Geometry: final body of the model. Coordinates: model frame, mm. A direction names the side the tool comes from. Give positions to 0.01 mm unless a question says otherwise; leave off trailing zeros. Loops run counter-clockwise (first coordinate to the right, second up) from the corner with the lowest first, then second, coordinate; pieces in that order, holes last. Notation, with made-up numbers: (61.5, 47) - (100.5, 47) arc R20 ccw to (100.5, 82) - close; hole circle Ø9 at (35, 1.25). An arc over 180 degrees is marked (long way). Answer in a Markdown table with one row per item.
from build123d import *

# Parameters (mm, degrees)
BOSS_EXTRUDE1_DEPTH = 265.3
SKETCH2_W           = 10
SKETCH2_H           = 44
BOSS_EXTRUDE2_DEPTH = 10
SKETCH3_W           = 381.110289958
SKETCH3_H           = 88.245673433
CUT_EXTRUDE1_DEPTH  = 27
SKETCH4_W           = 28
SKETCH4_H           = 7
BOSS_EXTRUDE3_DEPTH = 7


with BuildPart() as part:
    # Sketch1 → Boss-Extrude1 (new body)
    with BuildSketch(Plane(origin=(0, 0, 0), x_dir=(1, 0, 0), z_dir=(0, 1, 0))):
        Polygon((-51.505795374, 37), (-51.505795374, -18), (-41.505795374, -18), (-41.505795374, -37), (-38.505795374, -37), (-38.505795374, -22), (-35.205795374, -22), (-35.205795374, -37), (-32.205795374, -37), (-32.205795374, 37), align=None)
    extrude(amount=BOSS_EXTRUDE1_DEPTH)

    # Sketch2 → Boss-Extrude2 (add)
    with BuildSketch(Plane(origin=(0, 265.3, 0), x_dir=(1, 0, 0), z_dir=(0, 1, 0))):
        with Locations((-41.505795374, 15)):
            Rectangle(SKETCH2_W, SKETCH2_H)
    extrude(amount=BOSS_EXTRUDE2_DEPTH)

    # Sketch3 → Cut-Extrude1 (cut)
    with BuildSketch(Plane(origin=(-16.102897687, -16.102897687, 0), x_dir=(0, 0, -1), z_dir=(-0.7071067811865488, -0.7071067811865464, 0))):
        with Locations((41.438548882, -32.158306753)):
            Rectangle(SKETCH3_W, SKETCH3_H)
    extrude(amount=CUT_EXTRUDE1_DEPTH, mode=Mode.SUBTRACT)

    # Sketch4 → Boss-Extrude3 (add)
    with BuildSketch(Plane(origin=(-16.102897687, -16.102897687, 0), x_dir=(0, 0, 1), z_dir=(-0.7071067811865487, -0.7071067811865465, 0))):
        with Locations((-11, 40.567258056)):
            Rectangle(SKETCH4_W, SKETCH4_H)
    extrude(amount=BOSS_EXTRUDE3_DEPTH)


solid = part.part
Q1. First-contact query: pin 1 (5 mm diameter, centred on y = 118.5, z = -5, fed in from -X); pin 2 (6 mm diameter, centred on x = -45, z = -15, fed in from -Y); pin 3 (15 mm diameter, centred on y = 85, z = 26, fed in from -X); pin 4 (8 mm diameter, centred on x = -43.5, y = 268, fed in from +Z). Flat tips, straight axial feed; report the tip coordinate or a pass-through.
Check values:
| item | result |
|---|---|
| pin 1 | x = -51.51 |
| pin 2 | y = 5.16 |
| pin 3 | x = -41.51 |
| pin 4 | z = 37 |
Q2. Cut plane A-A (z = 30.5). Output: boundary loops of the cut face in (x, y), and give its area (3 significant figures).
Check values:
| item | result |
|---|---|
| outline | (-41.51, 9.3) - (-38.51, 6.3) - (-38.51, 265.3) - (-41.51, 265.3) - close; (-35.21, 3) - (-32.21, 0) - (-32.21, 265.3) - (-35.21, 265.3) - close |
| area | 1,560 mm² |
Q3. Cut plane B-B (z = -30.5). Output: boundary loops of the cut face in (x, y).
Check values:
| item | result |
|---|---|
| outline | (-51.51, 19.3) - (-32.21, 0) - (-32.21, 265.3) - (-36.51, 265.3) - (-36.51, 275.3) - (-46.51, 275.3) - (-46.51, 265.3) - (-51.51, 265.3) - close |
Q4. Material intervals for line 1 along X through (y, z) = (189, 22.5); line 2 along X through (y, z) = (178, -15); line 3 along X through (y, z) = (48, 21), sorted ascending.
Check values:
| item | result |
|---|---|
| line 1 | -41.51 to -38.51, -35.21 to -32.21 |
| line 2 | -51.51 to -32.21 |
| line 3 | -41.51 to -32.21 |
Q5. Cut plane C-C (y = 235). Output: boundary loops of the cut face in (x, z).
Check values:
| item | result |
|---|---|
| outline | (-51.51, -37) - (-32.21, -37) - (-32.21, 37) - (-35.21, 37) - (-35.21, 22) - (-38.51, 22) - (-38.51, 37) - (-41.51, 37) - (-41.51, 18) - (-51.51, 18) - close |
Q6. Cut plane D-D (z = -17.5). Output: boundary loops of the cut face in (x, y).
Check values:
| item | result |
|---|---|
| outline | (-52.21, 10.11) - (-47.26, 5.16) - (-42.31, 10.11) - (-32.21, 0) - (-32.21, 265.3) - (-36.51, 265.3) - (-36.51, 275.3) - (-46.51, 275.3) - (-46.51, 265.3) - (-51.51, 265.3) - (-51.51, 19.3) - (-47.26, 15.06) - close |
Q7. Draft query along Y for faces 1 (the flat face through (-44.75, 7.67, -11.2)), 2 (the flat face through (-41.721, 9.515, -7.704)), 3 (the flat face through (-36.506, 270, -15)). Return one class per face: pulls with the +Y half, pulls with the -Y half, needs draft (parallel to the pull), parting line crosses it, or undercut.
Check values:
| item | result |
|---|---|
| face 1 | pulls with the -Y half |
| face 2 | undercut |
| face 3 | needs draft |
Q8. Reachability of faces 4 (the flat face through (-46.506, 270, -15)), 5 (the flat face through (-49.7, 12.62, -11.2)), 6 (the flat face through (-42, 270, 7)) from +Z, -Z, +X, -X, +Y, -Y: full face, straight path, thin tool, end or side. Return the list, or none.
Check values:
| item | result |
|---|---|
| face 4 | +Z, -Z, -X, +Y |
| face 5 | +Z, -Z, -X |
| face 6 | +Z, +X, -X, +Y |
